from build123d import *

# Parameters (mm, degrees)
SKETCH1_R           = 12.5
SKETCH1_R_2         = 11.5
BOSS_EXTRUDE1_DEPTH = 60
CUT_EXTRUDE1_REACH  = 14.5
SKETCH2_R           = 1.5
SKETCH3_W           = 25.097425704
SKETCH3_H           = 25.030895612
BOSS_EXTRUDE2_DEPTH = 5
SKETCH4_R           = 7.5
CUT_EXTRUDE2_DEPTH  = 3


with BuildPart() as part:
    # Sketch1 → Boss-Extrude1 (new body)
    with BuildSketch(Plane(origin=(0, 0, 0), x_dir=(1, 0, 0), z_dir=(0, 1, 0))):
        Circle(SKETCH1_R)
        Circle(SKETCH1_R_2, mode=Mode.SUBTRACT)
    extrude(amount=BOSS_EXTRUDE1_DEPTH)

    # Sketch2 → Cut-Extrude1 (cut, up to next)
    with BuildSketch(Plane.XY, mode=Mode.PRIVATE) as cut_extrude1_sk1:
        with Locations((0, 6.62)):
            Circle(SKETCH2_R)
    cut_extrude1_tool1 = extrude(cut_extrude1_sk1.sketch, amount=CUT_EXTRUDE1_REACH, mode=Mode.PRIVATE) & part.part
    add(cut_extrude1_tool1.solids().sort_by_distance((0, 6.62, 0))[0], mode=Mode.SUBTRACT)

    # Sketch3 → Boss-Extrude2 (add)
    with BuildSketch(Plane(origin=(0, 60, 0), x_dir=(1, 0, 0), z_dir=(0, 1, 0))):
        Rectangle(SKETCH3_W, SKETCH3_H)
    extrude(amount=BOSS_EXTRUDE2_DEPTH)

    # Sketch4 → Cut-Extrude2 (cut)
    with BuildSketch(Plane(origin=(0, 65, 0), x_dir=(1, 0, 0), z_dir=(0, 1, 0))):
        Circle(SKETCH4_R)
    extrude(amount=-CUT_EXTRUDE2_DEPTH, mode=Mode.SUBTRACT)


solid = part.part
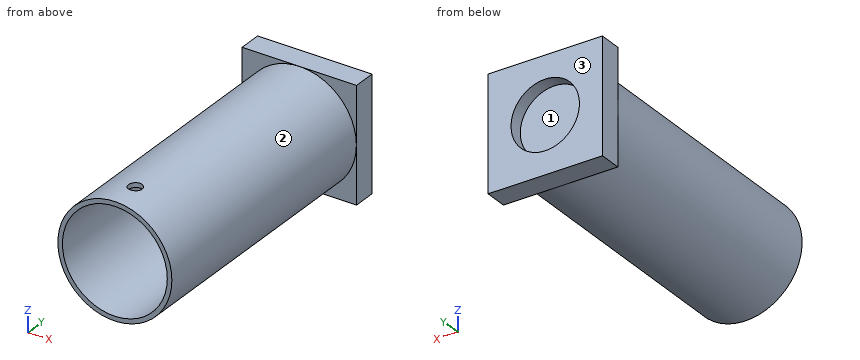
Work out the finished part from the listing and answer in its coordinate system (mm). Face numbers are marked on the shaded views. Coordinates: 2 decimals unless noted, no trailing zeros. Order: outer loops, then holes, each group sorted by start corner. A loop starts at its lowest first (then second) coordinate and runs counter-clockwise, first axis right, second up. Notation, with made-up numbers: (43, 34) - (99, 34) arc R13 ccw to (99, 40) - close; hole circle Ø10 at (24.5, -1). An arc over 180 degrees is marked (long way). Put each result on its own line as item: value. Start each with the question number.
1) Find section D-D (x = 6). Give the vertices of the cut face in (y, z).
2) Flat-ended cylindrical pins translate along their axes: pin 1 (1.5 mm diameter, centred on y = 27, z = -1.5, fed in from +X); pin 2 (3 mm diameter, centred on x = -2, z = -8, fed in from -Y); pin 3 (10 mm diameter, centred on x = 9, y = 22.5, fed in from +Z). Find the tip coordinate at first contact, or state that the pin passes through.
3) Find section C-C (y = 54). Give the vertices of the cut face in (x, z).
4) Find section B-B (z = 0). Give the vertices of the cut face in (x, y).
5) For a pull along Z with two mould halves and no side action, classify the marked faces 1, 2 and 3 as released by +Z, released by -Z, zero draft, split by the parting line, or undercut.
6) Find the intervals of material crossed by line 1 (Y direction, x = 0, z = 11.9); line 2 (X direction, y = 62.8, z = 0); line 3 (X direction, y = 32.5, z = 0), in increasing order. Write a range as from..to.
Results list:
1. outline: (0, -10.97) - (60, -10.97) - (60, -12.52) - (65, -12.52) - (65, -4.5) - (62, -4.5) - (62, 4.5) - (65, 4.5) - (65, 12.52) - (60, 12.52) - (60, 10.97) - (0, 10.97) - (0, 9.81) - (60, 9.81) - (60, -9.81) - (0, -9.81) - close
2. pin 1: stops at x = 12.48
2. pin 2: stops at y = 60
2. pin 3: stops at z = 11.84
3. outline: circle Ø25 at (0, 0); hole circle Ø23 at (0, 0)
4. outline: (-12.55, 60) - (-12.5, 60) - (-12.5, 0) - (-11.5, 0) - (-11.5, 60) - (11.5, 60) - (11.5, 0) - (12.5, 0) - (12.5, 60) - (12.55, 60) - (12.55, 65) - (7.5, 65) - (7.5, 62) - (-7.5, 62) - (-7.5, 65) - (-12.55, 65) - close
5. face 1: undercut
5. face 2: split by the parting line
5. face 3: zero draft
6. line 1: y = 0..5.12, 8.12..65
6. line 2: x = -12.55..-7.5, 7.5..12.55
6. line 3: x = -12.5..-11.5, 11.5..12.5
